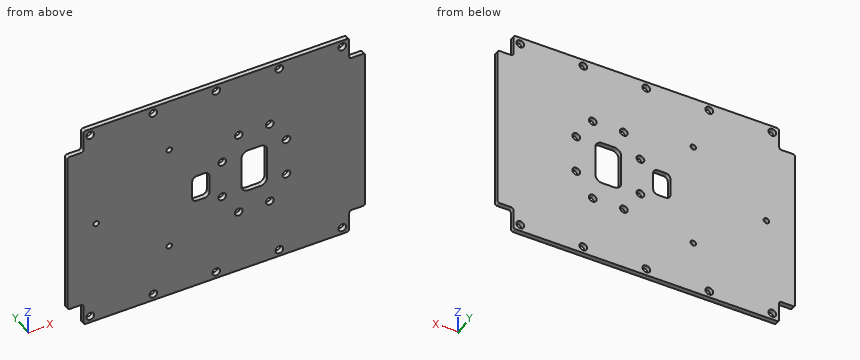
```python
from build123d import *

# Parameters (mm, degrees)
SKETCH_1_W             = 130
SKETCH_1_H             = 94.2
SM_BASE_FLANGE_1_DEPTH = 2
HOLE_WIZARD_M3_1_D     = 3.4
HOLE_WIZARD_M3_2_D     = 3.4
CUT_EXTRUDE_1_REACH    = 82.296
CUT_EXTRUDE_2_REACH    = 82.296
SKETCH_10_W            = 7.464918405
SKETCH_10_H            = 12
FILLET_2_R             = 2
HOLE_WIZARD_M2_1_D     = 2.4
CUT_EXTRUDE_3_DEPTH    = 81.295765766
FILLET_3_R             = 1


# Sheet-metal steps are written as plain solids
with BuildPart() as part:
    # Sketch 1 → 基体-法兰1 (new body)
    with BuildSketch(Plane(origin=(0, 0, 0), x_dir=(1, 0, 0), z_dir=(0, 1, 0))):
        Rectangle(SKETCH_1_W, SKETCH_1_H)
    extrude(amount=-SM_BASE_FLANGE_1_DEPTH)

    # M3 间隙孔1 (through all)
    with Locations(Plane(origin=(0, 0, 0), x_dir=(1, 0, 0), z_dir=(0, 1, 0))):
        with Locations((-55, -44.1), (-27.5, -44.1), (0, -44.1), (27.5, -44.1), (55, -44.1), (55, 44.1), (27.5, 44.1), (0, 44.1), (-27.5, 44.1), (-55, 44.1)):
            Hole(HOLE_WIZARD_M3_1_D / 2)

    # M3 间隙孔2 (through all)
    with Locations(Plane(origin=(0, 0, 0), x_dir=(1, 0, 0), z_dir=(0, 1, 0))):
        with Locations((2.567531914, -8.425296044), (2.567531914, 8.425296044), (9.795, 18.75), (23.395, 18.75), (30.622468086, 8.425296044), (30.622468086, -8.425296044), (23.395, -18.75), (9.795, -18.75)):
            Hole(HOLE_WIZARD_M3_2_D / 2)

    # 草图8 → 切除-拉伸1 (cut, up to next)
    with BuildSketch(Plane(origin=(0, 0, 0), x_dir=(1, 0, 0), z_dir=(0, 1, 0)), mode=Mode.PRIVATE) as cut_extrude_1_sk1:
        with BuildLine():
            Line((19.22, 9.75), (13.97, 9.75))
            ThreePointArc((13.97, 9.75), (11.848679656, 8.871320344), (10.97, 6.75))
            Line((10.97, 6.75), (10.97, -6.75))
            ThreePointArc((10.97, -6.75), (11.848679656, -8.871320344), (13.97, -9.75))
            Line((13.97, -9.75), (19.22, -9.75))
            ThreePointArc((19.22, -9.75), (21.341320344, -8.871320344), (22.22, -6.75))
            Line((22.22, -6.75), (22.22, 6.75))
            ThreePointArc((22.22, 6.75), (21.341320344, 8.871320344), (19.22, 9.75))
        make_face()
    cut_extrude_1_tool1 = extrude(cut_extrude_1_sk1.sketch, amount=-CUT_EXTRUDE_1_REACH, mode=Mode.PRIVATE) & part.part
    add(cut_extrude_1_tool1.solids().sort_by_distance((16.595, 0, 0))[0], mode=Mode.SUBTRACT)

    # 草图10 → 切除-拉伸2 (cut, up to next)
    with BuildSketch(Plane(origin=(0, 0, 0), x_dir=(1, 0, 0), z_dir=(0, 1, 0)), mode=Mode.PRIVATE) as cut_extrude_2_sk1:
        with Locations((-6.762459203, 0)):
            Rectangle(SKETCH_10_W, SKETCH_10_H)
    cut_extrude_2_tool1 = extrude(cut_extrude_2_sk1.sketch, amount=-CUT_EXTRUDE_2_REACH, mode=Mode.PRIVATE) & part.part
    add(cut_extrude_2_tool1.solids().sort_by_distance((-6.762459, 0, 0))[0], mode=Mode.SUBTRACT)

    # 圆角2
    fillet_2_edges = [part.edges().sort_by_distance(p)[0] for p in [
        (-10.494918405, -1, 6),
        (-10.494918405, -1, -6),
        (-3.03, -1, -6),
        (-3.03, -1, 6),
    ]]
    fillet(fillet_2_edges, radius=FILLET_2_R)

    # M2 间隙孔1 (through all)
    with Locations(Plane(origin=(0, 0, 0), x_dir=(1, 0, 0), z_dir=(0, 1, 0))):
        with Locations((-20.514677996, 23.3999532), (-20.514677996, -23.3999532), (-52.431517644, 0)):
            Hole(HOLE_WIZARD_M2_1_D / 2)

    # 草图14 → 切除-拉伸3 (cut, through all)
    with BuildSketch(Plane(origin=(0, 0, 0), x_dir=(1, 0, 0), z_dir=(0, 1, 0))):
        with BuildLine():
            Line((-65, 47.1), (-58, 47.1))
            Line((-58, 47.1), (-58, 38.1))
            ThreePointArc((-58, 38.1), (-58.292893219, 37.392893219), (-59, 37.1))
            Line((-59, 37.1), (-65, 37.1))
            Line((-65, 37.1), (-65, 47.1))
        make_face()
        with BuildLine():
            Line((-58, -47.1), (-58, -38.1))
            ThreePointArc((-58, -38.1), (-58.292893219, -37.392893219), (-59, -37.1))
            Line((-59, -37.1), (-65, -37.1))
            Line((-65, -37.1), (-65, -47.1))
            Line((-65, -47.1), (-58, -47.1))
        make_face()
        with BuildLine():
            Line((65, -47.1), (58, -47.1))
            Line((58, -47.1), (58, -38.1))
            ThreePointArc((58, -38.1), (58.292893219, -37.392893219), (59, -37.1))
            Line((59, -37.1), (65, -37.1))
            Line((65, -37.1), (65, -47.1))
        make_face()
        with BuildLine():
            Line((58, 47.1), (58, 38.1))
            ThreePointArc((58, 38.1), (58.292893219, 37.392893219), (59, 37.1))
            Line((59, 37.1), (65, 37.1))
            Line((65, 37.1), (65, 47.1))
            Line((65, 47.1), (58, 47.1))
        make_face()
    extrude(amount=-CUT_EXTRUDE_3_DEPTH, mode=Mode.SUBTRACT)

    # 圆角3
    fillet_3_edges = [part.edges().sort_by_distance(p)[0] for p in [
        (58, -1, -47.1),
        (65, -1, -37.1),
        (65, -1, 37.1),
        (58, -1, 47.1),
        (-58, -1, 47.1),
        (-65, -1, 37.1),
        (-65, -1, -37.1),
        (-58, -1, -47.1),
    ]]
    fillet(fillet_3_edges, radius=FILLET_3_R)


solid = part.part
```
Input: part model. Units: mm. Frame: model coordinates. Give positions to 0.01 mm unless a question says otherwise; leave off trailing zeros. Loops run counter-clockwise (first coordinate to the right, second up) from the corner with the lowest first, then second, coordinate; pieces in that order, holes last. Notation, with made-up numbers: M -1.5,81.25 L 31.5,81.25 A22 ccw 31.5,92.25 Z; hole C 64.5,0.25 d2. An arc over 180 degrees is marked long. Answer as CSV lines item,"result". Start each with the question number.
1. Section C-C on z = 44.1. Return loops of the section in (x, y), plus the area to 3 significant figures.
2. Pin query (flat end, axial travel): P1, Ø2.5, axis at x = 27.5, z = -44.1, coming from the -Y side; P2, Ø1, axis at x = 62, y = -1, coming from the -Z side. Return the tip coordinate at first contact, or that it passes through.
3. Section D-D on y = -0.7. State how many separate pieces and enclosed holes the cut face has, plus the area to 3 significant figures.
4. Section B-B on z = 18.75. Return loops of the section in (x, y) (3 decimals).
5. Section A-A on x = 27.5. Return loops of the section in (y, z), plus the area to 3 significant figures.
6. Line query: L1, parallel to Z at x = -27.5, y = -1.15; L2, parallel to Z at x = 23.5, y = -0.95; L3, parallel to X at y = -0.7, z = 44.1. Output: solid intervals per line, ascending.
Computed values:
1,outline,"M -58,-2 L -56.7,-2 L -56.7,0 L -58,0 Z; M -53.3,-2 L -29.2,-2 L -29.2,0 L -53.3,0 Z; M -25.8,-2 L -1.7,-2 L -1.7,0 L -25.8,0 Z; M 1.7,-2 L 25.8,-2 L 25.8,0 L 1.7,0 Z; M 29.2,-2 L 53.3,-2 L 53.3,0 L 29.2,0 Z; M 56.7,-2 L 58,-2 L 58,0 L 56.7,0 Z"
1,area,"198 mm²"
2,P1,"passes through"
2,P2,"stops at z = -37.1"
3,separate pieces,"1"
3,enclosed holes,"23"
3,area,"11,500 mm²"
4,outline,"M -65,-2 L 8.095,-2 L 8.095,0 L -65,0 Z; M 11.495,-2 L 21.695,-2 L 21.695,0 L 11.495,0 Z; M 25.095,-2 L 65,-2 L 65,0 L 25.095,0 Z"
5,outline,"M -2,-47.1 L 0,-47.1 L 0,-45.8 L -2,-45.8 Z; M -2,-42.4 L 0,-42.4 L 0,42.4 L -2,42.4 Z; M -2,45.8 L 0,45.8 L 0,47.1 L -2,47.1 Z"
5,area,"175 mm²"
6,L1,"z = -47.1 to -45.8, -42.4 to 42.4, 45.8 to 47.1"
6,L2,"z = -47.1 to -20.45, -17.05 to 17.05, 20.45 to 47.1"
6,L3,"x = -58 to -56.7, -53.3 to -29.2, -25.8 to -1.7, 1.7 to 25.8, 29.2 to 53.3, 56.7 to 58"
